```python
from build123d import *

# Parameters (mm, degrees)
SKETCH2_W           = 110
SKETCH2_H           = 15
BOSS_EXTRUDE1_DEPTH = 3.25
CAVITY1_START       = -2.5
CAVITY1_DEPTH       = 2.5
CAVITY1_START_2     = -1.5
CAVITY1_2_DEPTH     = 4.75
CAVITY1_3_DEPTH     = 1.5
CUT_EXTRUDE1_START  = -5.75
CUT_EXTRUDE1_DEPTH  = 5.75
CUT_EXTRUDE2_START  = -1
CUT_EXTRUDE2_DEPTH  = 1
CUT_EXTRUDE3_START  = -0.2
CUT_EXTRUDE3_DEPTH  = 2.7
CUT_EXTRUDE4_REACH  = 57.888
SKETCH9_W           = 88
SKETCH9_H           = 15
CUT_EXTRUDE5_DEPTH  = 56.888281419


# Read off the part's stored shape, not the designer's step: Cavity1
with BuildPart() as part:
    # Sketch2 → Boss-Extrude1 (new, symmetric)
    with BuildSketch(Plane(origin=(0, 0, 0), x_dir=(1, 0, 0), z_dir=(0, 1, 0))):
        Rectangle(SKETCH2_W, SKETCH2_H)
    extrude(amount=BOSS_EXTRUDE1_DEPTH, both=True)

    # Cavity1 outline → Cavity1 (cut)
    with BuildSketch(Plane(origin=(0, 0, 0), x_dir=(1, 0, 0), z_dir=(0, 1, 0)).offset(CAVITY1_START)):
        with BuildLine():
            ThreePointArc((-55, 2.875), (-52.125, 0), (-55, -2.875))
            Line((-55, -2.875), (-55, -3.425))
            ThreePointArc((-55, -3.425), (-51.575, 0), (-55, 3.425))
            Line((-55, 3.425), (-55, 2.875))
        make_face()
        with BuildLine():
            Line((-55, 6.05), (-55, 4.5))
            ThreePointArc((-55, 4.5), (-50.5, 0), (-55, -4.5))
            Line((-55, -4.5), (-55, -6.05))
            ThreePointArc((-55, -6.05), (-52.834647835, -5.649225611), (-50.956177551, -4.5))
            Line((-50.956177551, -4.5), (-38.326846611, -2.75))
            ThreePointArc((-38.326846611, -2.75), (-35.931628674, 0), (-38.326846611, 2.75))
            Line((-38.326846611, 2.75), (-50.956177551, 4.5))
            ThreePointArc((-50.956177551, 4.5), (-52.834647835, 5.649225611), (-55, 6.05))
        make_face()
    extrude(amount=CAVITY1_DEPTH, mode=Mode.SUBTRACT)

    # Cavity1 2 outline → Cavity1 2 (cut)
    with BuildSketch(Plane(origin=(0, 0, 0), x_dir=(1, 0, 0), z_dir=(0, 1, 0)).offset(CAVITY1_START_2)):
        with BuildLine():
            ThreePointArc((-55, 3), (-52, 0), (-55, -3))
            Line((-55, -3), (-55, -4.375))
            ThreePointArc((-55, -4.375), (-50.625, 0), (-55, 4.375))
            Line((-55, 4.375), (-55, 3))
        make_face()
    extrude(amount=CAVITY1_2_DEPTH, mode=Mode.SUBTRACT)

    # Cavity1 3 outline → Cavity1 3 (cut)
    with BuildSketch(Plane(origin=(0, 0, 0), x_dir=(1, 0, 0), z_dir=(0, 1, 0)).offset(CAVITY1_START_2)):
        with BuildLine():
            Line((-55, 2.875), (-55, 1.5))
            ThreePointArc((-55, 1.5), (-53.5, 0), (-55, -1.5))
            Line((-55, -1.5), (-55, -2.875))
            ThreePointArc((-55, -2.875), (-52.125, 0), (-55, 2.875))
        make_face()
        with BuildLine():
            Line((-55, 4.5), (-55, 4.375))
            ThreePointArc((-55, 4.375), (-50.625, 0), (-55, -4.375))
            Line((-55, -4.375), (-55, -4.5))
            ThreePointArc((-55, -4.5), (-50.5, 0), (-55, 4.5))
        make_face()
    extrude(amount=CAVITY1_3_DEPTH, mode=Mode.SUBTRACT)

    # Sketch4 → Cut-Extrude1 (cut)
    with BuildSketch(Plane(origin=(0, 3.25, 0), x_dir=(1, 0, 0), z_dir=(0, 1, 0)).offset(CUT_EXTRUDE1_START)):
        with BuildLine():
            Line((-55, 3), (-55, -3))
            ThreePointArc((-55, -3), (-52, 0), (-55, 3))
        make_face()
    extrude(amount=CUT_EXTRUDE1_DEPTH, mode=Mode.SUBTRACT)

    # Sketch6 → Cut-Extrude2 (cut)
    with BuildSketch(Plane(origin=(0, -1.5, 0), x_dir=(1, 0, 0), z_dir=(0, 1, 0)).offset(CUT_EXTRUDE2_START)):
        with BuildLine():
            Line((-55, 4.5), (-55, 3.425))
            ThreePointArc((-55, 3.425), (-51.575, 0), (-55, -3.425))
            Line((-55, -3.425), (-55, -4.5))
            ThreePointArc((-55, -4.5), (-50.5, 0), (-55, 4.5))
        make_face()
    extrude(amount=CUT_EXTRUDE2_DEPTH, mode=Mode.SUBTRACT)

    # Sketch7 → Cut-Extrude3 (cut)
    with BuildSketch(Plane(origin=(0, -2.5, 0), x_dir=(1, 0, 0), z_dir=(0, 1, 0)).offset(CUT_EXTRUDE3_START)):
        with BuildLine():
            Line((-38.25821916, 3.24526788), (-50.739154033, 4.974705182))
            ThreePointArc((-50.739154033, 4.974705182), (-52.964952838, 6.225839947), (-55.5, 6.530888148))
            Line((-55.5, 6.530888148), (-55.5, -6.530888148))
            ThreePointArc((-55.5, -6.530888148), (-52.964952838, -6.225839947), (-50.739154033, -4.974705182))
            Line((-50.739154033, -4.974705182), (-38.25821916, -3.24526788))
            ThreePointArc((-38.25821916, -3.24526788), (-35.431628674, 0), (-38.25821916, 3.24526788))
        make_face()
    extrude(amount=CUT_EXTRUDE3_DEPTH, mode=Mode.SUBTRACT)

    # Sketch8 → Cut-Extrude4 (cut, up to next)
    with BuildSketch(Plane(origin=(0, 3.25, 0), x_dir=(1, 0, 0), z_dir=(0, 1, 0)), mode=Mode.PRIVATE) as cut_extrude4_sk1:
        with BuildLine():
            ThreePointArc((-55, 4.375), (-50.625, 0), (-55, -4.375))
            Line((-55, -4.375), (-55, -4.875))
            ThreePointArc((-55, -4.875), (-50.125, 0), (-55, 4.875))
            Line((-55, 4.875), (-55, 4.375))
        make_face()
    cut_extrude4_tool1 = extrude(cut_extrude4_sk1.sketch, amount=-CUT_EXTRUDE4_REACH, mode=Mode.PRIVATE) & part.part
    add(cut_extrude4_tool1.solids().sort_by_distance((-50.515992, 3.25, 0))[0], mode=Mode.SUBTRACT)

    # Sketch9 → Cut-Extrude5 (cut, through all)
    with BuildSketch(Plane(origin=(0, 3.25, 0), x_dir=(1, 0, 0), z_dir=(0, 1, 0))):
        with Locations((11, 0)):
            Rectangle(SKETCH9_W, SKETCH9_H)
    extrude(amount=-CUT_EXTRUDE5_DEPTH, mode=Mode.SUBTRACT)


solid = part.part
```
Geometry: final body of the model. Coordinates: model frame, mm. A direction names the side the tool comes from. Round coordinates to 2 decimals unless told otherwise and drop trailing zeros. Order: outer loops, then holes, each group sorted by start corner. A loop starts at its lowest first (then second) coordinate and runs counter-clockwise, first axis right, second up. Notation, with made-up numbers: M 17,26 L 51,26 A19 ccw 51,57 Z; hole C 25,6.5 d6. An arc over 180 degrees is marked long. One line per item, written item: value.
(1) Cut plane B-B (x = -49.75). Return the cut outline in (y, z).
Result sheet:
outline: M -3.25,-7.5 L 3.25,-7.5 L 3.25,7.5 L -3.25,7.5 Z; hole M -2.7,-4.84 L 0,-4.84 L 0,4.84 L -2.7,4.84 Z
(2) Line query: probe 1 along Y at (x, z) = (-45.75, 1.5); probe 2 along Z at (x, y) = (-51.75, 0.75); probe 3 along Z at (x, y) = (-42, -2.25). Output: solid intervals per line, ascending. Write a range as [from, to].
Result sheet:
probe 1: [-3.25, -2.7], [0, 3.25]
probe 2: [-7.5, -3.63], [3.63, 7.5]
probe 3: [-7.5, -3.76], [3.76, 7.5]
(3) Pull-direction query (Y, two-part tool) for faces 1 (the flat face through (-44, 3.25, 0)), 2 (the cylindrical face through (-52.759, -1.369, 6.155)), 3 (the flat face through (-44, 0, -7.5)); classes: pulls with the +Y half, pulls with the -Y half, needs draft (parallel to the pull), parting line crosses it, or undercut.
Result sheet:
face 1: pulls with the +Y half
face 2: undercut
face 3: needs draft
(4) Reachability of faces 4 (the flat face through (-48, -2.7, 0)), 5 (the flat face through (-44, 0, 7.5)), 6 (the cylindrical face through (-50.126, 1.648, 0.107)) from +Z, -Z, +X, -X, +Y, -Y: full face, straight path, thin tool, end or side. Return the list, or none.
Result sheet:
face 4: -X
face 5: +Z, +X, -X, +Y, -Y
face 6: -X, +Y
(5) Pin query (flat end, axial travel): P1, Ø1.5, axis at y = 0.5, z = -1, coming from the -X side. Return the tip coordinate at first contact, or that it passes through.
Result sheet:
P1: x = -50.45
(6) Cut plane A-A (z = 0). Return the cut outline in (x, y) (3 decimals).
Result sheet:
outline: M -55,-3.25 L -33,-3.25 L -33,3.25 L -50.125,3.25 L -50.125,0 L -35.432,0 L -35.432,-2.7 L -55,-2.7 Z
(7) Cut plane C-C (y = -0.5). Return the cut outline in (x, z), and give its area (3 significant figures).
Result sheet:
outline: M -55,-7.5 L -33,-7.5 L -33,7.5 L -55,7.5 L -55,6.55 A6.55 cw -50.74,4.97 L -38.26,3.25 A3.28 cw -38.26,-3.25 L -50.74,-4.97 A6.55 cw -55,-6.55 Z
area: 162 mm2
(8) Cut plane D-D (z = -4.25). Return the cut outline in (x, y), and give its area (3 significant figures).
Result sheet:
outline: M -55,-3.25 L -33,-3.25 L -33,3.25 L -52.61,3.25 L -52.61,0 L -45.51,0 L -45.51,-2.7 L -55,-2.7 Z
area: 110 mm2
